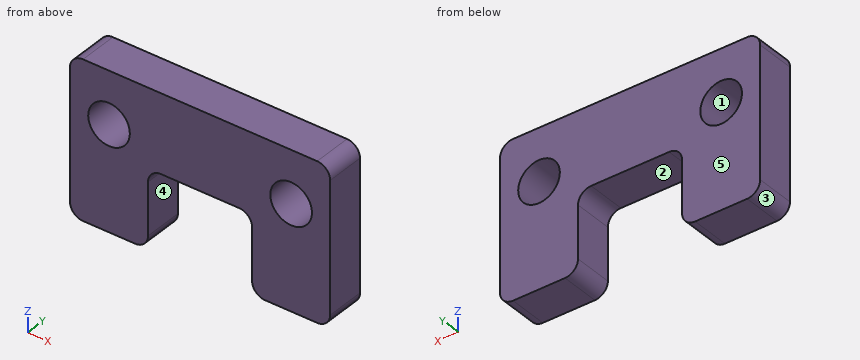
```python
from build123d import *

# Parameters (mm, degrees)
SKETCH_1_R      = 1.6
EXTRUDE_1_DEPTH = 3
FILLET_1_R      = 1


with BuildPart() as part:
    # 草图1 → 凸台-拉伸1 (new body)
    with BuildSketch(Plane(origin=(0, 0, 0), x_dir=(1, 0, 0), z_dir=(0, 1, 0))):
        Polygon((-10, 0), (10, 0), (10, 12), (4, 12), (4, 6), (-4, 6), (-4, 12), (-10, 12), align=None)
        with Locations(Location((7, 4, 0), (0, 0, 270))):
            Circle(SKETCH_1_R, mode=Mode.SUBTRACT)
        with Locations(Location((-7, 4, 0), (0, 0, 90))):
            Circle(SKETCH_1_R, mode=Mode.SUBTRACT)
    extrude(amount=EXTRUDE_1_DEPTH)

    # 圆角1
    fillet_1_edges = [part.edges().sort_by_distance(p)[0] for p in [
        (-4, 1.5, -12),
        (-4, 1.5, -6),
        (4, 1.5, -6),
        (4, 1.5, -12),
        (10, 1.5, -12),
        (10, 1.5, 0),
        (-10, 1.5, 0),
        (-10, 1.5, -12),
    ]]
    fillet(fillet_1_edges, radius=FILLET_1_R)


solid = part.part
```
Here's how the part is built. I have some questions about the finished solid (model axes, mm). Face numbers are marked on the shaded views. A direction names the side the tool comes from. Coordinates: 2 decimals unless noted, no trailing zeros. Order: outer loops, then holes, each group sorted by start corner. A loop starts at its lowest first (then second) coordinate and runs counter-clockwise, first axis right, second up. Notation, with made-up numbers: (-29.75, 36) - (-18.75, 36) arc R22 cw to (-18.75, 64) - close; hole circle Ø9 at (73, 38). An arc over 180 degrees is marked (long way). One line per question, with ' | ' between items.
(1) Will this pin go through, and if not, where does the flat tip stop? pin 1 (1.9 mm diameter, centred on x = 7, z = -4, fed in from +Y).
Report:
pin 1: passes through
(2) Suppose I cut it at B-B on z = -4. List the corners of the cut face in (x, y) for me, and give its area (3 significant figures).
Report:
outline: (-10, 0) - (-8.6, 0) - (-8.6, 3) - (-10, 3) - close; (-5.4, 0) - (5.4, 0) - (5.4, 3) - (-5.4, 3) - close; (8.6, 0) - (10, 0) - (10, 3) - (8.6, 3) - close | area: 40.8 mm2
(3) Suppose I cut it at C-C on y = 0.6. List the corners of the cut face in (x, z) for me.
Report:
outline: (-10, -11) arc R1 ccw to (-9, -12) - (-5, -12) arc R1 ccw to (-4, -11) - (-4, -7) arc R1 cw to (-3, -6) - (3, -6) arc R1 cw to (4, -7) - (4, -11) arc R1 ccw to (5, -12) - (9, -12) arc R1 ccw to (10, -11) - (10, -1) arc R1 ccw to (9, 0) - (-9, 0) arc R1 ccw to (-10, -1) - close; hole circle Ø3.2 at (-7, -4); hole circle Ø3.2 at (7, -4)
(4) For the marked faces 1 and 2, which set-ups out of +Z, -Z, +X, -X, +Y, -Y let a thin tool reach every point of the face, with its end or its side?
Report:
face 1: +Y, -Y | face 2: -Z, +Y, -Y
(5) If I drill on L1, parallel to X at y = 2, z = -4; L2, parallel to X at y = 1.2, z = -11; L3, parallel to Z at x = -7, y = 2.25, over which ranges is the centre line in solid material (lowest first)?
Report:
L1: x = -10 to -8.6, -5.4 to 5.4, 8.6 to 10 | L2: x = -10 to -4, 4 to 10 | L3: z = -12 to -5.6, -2.4 to 0
(6) If we mould it in two halves opening along X, with no side actions, what happens to the marked faces 3, 4 and 5? For each: pulls with the +X half, pulls with the -X half, needs draft (parallel to the pull), parting line crosses it, or undercut.
Report:
face 3: pulls with the -X half | face 4: undercut | face 5: needs draft
(7) Suppose I cut it at D-D on z = -7.5. List the corners of the cut face in (x, y) for me.
Report:
outline: (-10, 0) - (-4, 0) - (-4, 3) - (-10, 3) - close; (4, 0) - (10, 0) - (10, 3) - (4, 3) - close
(8) Suppose I cut it at A-A on x = -7. List the corners of the cut face in (y, z) for me.
Report:
outline: (0, -12) - (3, -12) - (3, -5.6) - (0, -5.6) - close; (0, -2.4) - (3, -2.4) - (3, 0) - (0, 0) - close
